Job drawing, mm, ordinate dimensions from the low corner. One solid piece. A direction names the side the tool comes from. Give positions to 0.01 mm unless a question says otherwise; leave off trailing zeros. Write each loop counter-clockwise with the first axis right and the second up, starting at its lowest first coordinate (ties: lowest second). Pieces come first, ordered by that corner, then holes. Notation, with made-up numbers: (53.5, -37.75) - (77.5, -37.75) arc R32 ccw to (77.5, -7.75) - close; hole circle Ø7 at (-27.75, 32.25). An arc over 180 degrees is marked (long way). Answer in a Markdown table with one row per item. Add a question column.
1. Band-saw the part on C-C on z = 29.5. Write the cut outline in (x, y), plus the area to 3 significant figures.
2. Which spindle directions (+Z, -Z, +X, -X, +Y, -Y) get a long thin tool onto all of the face, cutting with end or side? Do the marked faces 1, 2, 3 and 4. Say none if no direction does.
3. Drop flat-ended pins along their axis: pin 1 Ø3 at (x, z) = (49.5, 21) entering from -Y; pin 2 Ø2 at (y, z) = (11, 5.5) entering from -X; pin 3 Ø9 at (y, z) = (18, 8) entering from +X; pin 4 Ø5 at (x, y) = (74.5, 18.5) entering from -Z. Give the stop position or say it passes through.
4. Probe line 1 along Z through (x, y) = (22, 11.75); line 2 along X through (y, z) = (13, 6.5); line 3 along Y through (x, z) = (77, 22.5). List the from-to ranges inside material, lowest first.
5. Band-saw the part on B-B on x = 58. Write the cut outline in (y, z).
6. Band-saw the part on D-D on z = 5. Write the cut outline in (x, y).
7. Band-saw the part on A-A on y = 7. Write the cut outline in (x, z).
8. Pull direction Z, two halves, no side cores. Call the marked faces 5, 6 and 7: released by +Z, released by -Z, zero draft, split by the parting line, or undercut.
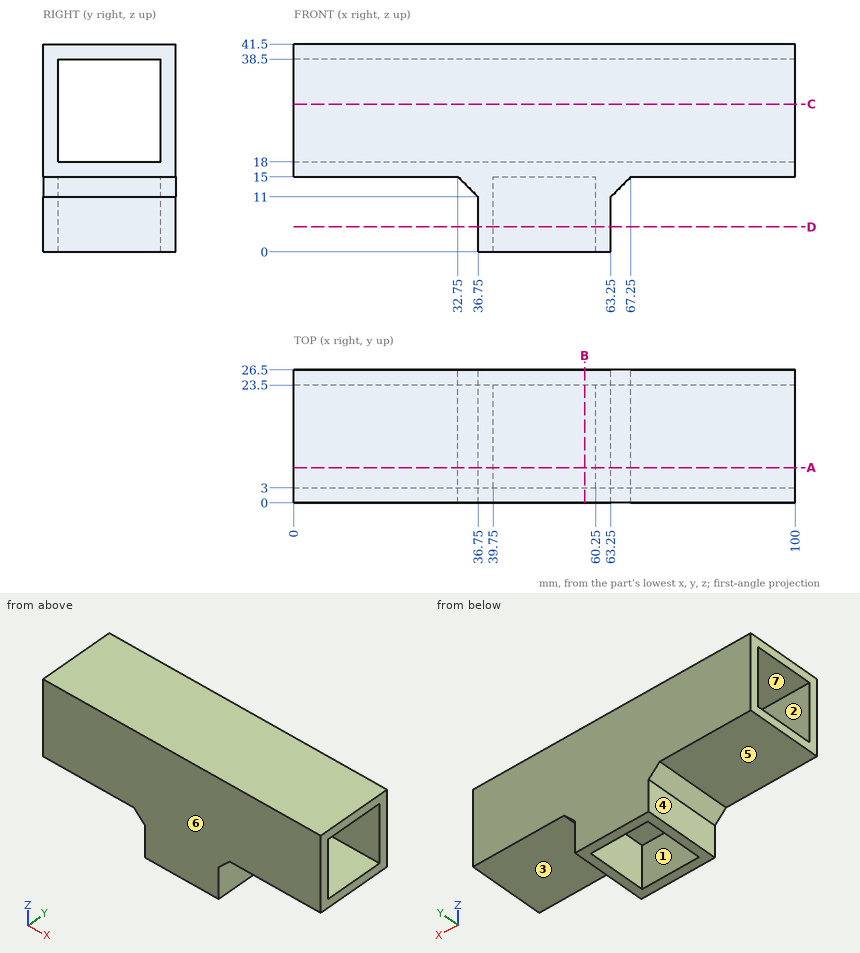
Values:
| question | item | result |
|---|---|---|
| 1 | outline | (0, 0) - (100, 0) - (100, 3) - (0, 3) - close; (0, 23.5) - (100, 23.5) - (100, 26.5) - (0, 26.5) - close |
| 1 | area | 600 mm² |
| 2 | face 1 | -Z |
| 2 | face 2 | +X, -X |
| 2 | face 3 | -Z, +X, +Y, -Y |
| 2 | face 4 | -Z, -X, +Y, -Y |
| 3 | pin 1 | stops at y = 0 |
| 3 | pin 2 | stops at x = 36.75 |
| 3 | pin 3 | stops at x = 64.75 |
| 3 | pin 4 | stops at z = 15 |
| 4 | line 1 | z = 15 to 18, 38.5 to 41.5 |
| 4 | line 2 | x = 36.75 to 39.75, 60.25 to 63.25 |
| 4 | line 3 | y = 0 to 3, 23.5 to 26.5 |
| 5 | outline | (0, 0) - (3, 0) - (3, 15) - (23.5, 15) - (23.5, 0) - (26.5, 0) - (26.5, 41.5) - (0, 41.5) - close; hole (3, 18) - (23.5, 18) - (23.5, 38.5) - (3, 38.5) - close |
| 6 | outline | (36.75, 0) - (63.25, 0) - (63.25, 26.5) - (36.75, 26.5) - close; hole (39.75, 3) - (60.25, 3) - (60.25, 23.5) - (39.75, 23.5) - close |
| 7 | outline | (0, 15) - (32.75, 15) - (36.75, 11) - (36.75, 0) - (39.75, 0) - (39.75, 15) - (60.25, 15) - (60.25, 0) - (63.25, 0) - (63.25, 11) - (67.25, 15) - (100, 15) - (100, 18) - (0, 18) - close; (0, 38.5) - (100, 38.5) - (100, 41.5) - (0, 41.5) - close |
| 8 | face 5 | released by -Z |
| 8 | face 6 | zero draft |
| 8 | face 7 | undercut |
